```python
from build123d import *

# Parameters (mm, degrees)
SKETCH1_W           = 71.6
SKETCH1_H           = 161
SKETCH1_W_2         = 68
SKETCH1_H_2         = 30.04
BOSS_EXTRUDE1_DEPTH = 1.8
SKETCH1_6_W         = 71.6
SKETCH1_6_H         = 161
SKETCH1_6_W_2       = 68
SKETCH1_6_H_2       = 30.04
BOSS_EXTRUDE2_DEPTH = 20.1
FILLET3_SIZE        = 15
FILLET3_SIZE_2      = 10
FILLET4_R           = 15
FILLET5_SIZE        = 20
FILLET5_SIZE_2      = 15
FILLET6_SIZE        = 10
FILLET6_SIZE_2      = 15
FILLET7_SIZE        = 10
FILLET7_SIZE_2      = 15


with BuildPart() as part:
    # Sketch1 → Boss-Extrude1 (new body)
    # profile 1 of 6: a face of its own
    with BuildSketch(Plane(origin=(0, 0, 0), x_dir=(1, 0, 0), z_dir=(0, 1, 0))):
        with Locations((35.8, 80.5)):
            Rectangle(SKETCH1_W, SKETCH1_H)
        with Locations((35.8, 48.66)):
            Rectangle(SKETCH1_W_2, SKETCH1_H_2, mode=Mode.SUBTRACT)
        with Locations((35.8, 16.82)):
            Rectangle(SKETCH1_W_2, SKETCH1_H_2, mode=Mode.SUBTRACT)
        with Locations((35.8, 80.5)):
            Rectangle(SKETCH1_W_2, SKETCH1_H_2, mode=Mode.SUBTRACT)
        with Locations((35.8, 112.34)):
            Rectangle(SKETCH1_W_2, SKETCH1_H_2, mode=Mode.SUBTRACT)
        with Locations((35.8, 144.18)):
            Rectangle(SKETCH1_W_2, SKETCH1_H_2, mode=Mode.SUBTRACT)
    # profile 2 of 6: a face of its own
    with BuildSketch(Plane(origin=(0, 0, 0), x_dir=(1, 0, 0), z_dir=(0, 1, 0))):
        with Locations((35.8, 144.18)):
            Rectangle(SKETCH1_W_2, SKETCH1_H_2)
    # profile 3 of 6: a face of its own
    with BuildSketch(Plane(origin=(0, 0, 0), x_dir=(1, 0, 0), z_dir=(0, 1, 0))):
        with Locations((35.8, 112.34)):
            Rectangle(SKETCH1_W_2, SKETCH1_H_2)
    # profile 4 of 6: a face of its own
    with BuildSketch(Plane(origin=(0, 0, 0), x_dir=(1, 0, 0), z_dir=(0, 1, 0))):
        with Locations((35.8, 80.5)):
            Rectangle(SKETCH1_W_2, SKETCH1_H_2)
    # profile 5 of 6: a face of its own
    with BuildSketch(Plane(origin=(0, 0, 0), x_dir=(1, 0, 0), z_dir=(0, 1, 0))):
        with Locations((35.8, 48.66)):
            Rectangle(SKETCH1_W_2, SKETCH1_H_2)
    # profile 6 of 6: a face of its own
    with BuildSketch(Plane(origin=(0, 0, 0), x_dir=(1, 0, 0), z_dir=(0, 1, 0))):
        with Locations((35.8, 16.82)):
            Rectangle(SKETCH1_W_2, SKETCH1_H_2)
    extrude(amount=-BOSS_EXTRUDE1_DEPTH)

    # Sketch1<6> → Boss-Extrude2 (add)
    with BuildSketch(Plane(origin=(0, 0, 0), x_dir=(1, 0, 0), z_dir=(0, 1, 0))):
        with Locations((35.8, 80.5)):
            Rectangle(SKETCH1_6_W, SKETCH1_6_H)
        with Locations((35.8, 16.82)):
            Rectangle(SKETCH1_6_W_2, SKETCH1_6_H_2, mode=Mode.SUBTRACT)
        with Locations((35.8, 80.5)):
            Rectangle(SKETCH1_6_W_2, SKETCH1_6_H_2, mode=Mode.SUBTRACT)
        with Locations((35.8, 48.66)):
            Rectangle(SKETCH1_6_W_2, SKETCH1_6_H_2, mode=Mode.SUBTRACT)
        with Locations((35.8, 112.34)):
            Rectangle(SKETCH1_6_W_2, SKETCH1_6_H_2, mode=Mode.SUBTRACT)
        with Locations((35.8, 144.18)):
            Rectangle(SKETCH1_6_W_2, SKETCH1_6_H_2, mode=Mode.SUBTRACT)
    extrude(amount=BOSS_EXTRUDE2_DEPTH)

    # Fillet3
    # an asymmetric fillet: 15, 10 mm, written as the material it adds along each edge
    with BuildSketch(Plane(origin=(69.8, 0, -159.2), x_dir=(0, 1, 0), z_dir=(0, 0, 1))) as fillet3_piece_1_section:
        with BuildLine():
            Bezier((FILLET3_SIZE, 0), (0, 0), (0, FILLET3_SIZE_2), weights=[1, 0.707106781, 1])
            Line((0, FILLET3_SIZE_2), (0, 0))
            Line((0, 0), (FILLET3_SIZE, 0))
        make_face()
    fillet3_piece_1 = extrude(amount=67.54, mode=Mode.PRIVATE)
    fillet3_piece_1 = split(fillet3_piece_1, bisect_by=Plane(origin=(67.566321176, 3.350519055, -127.36), z_dir=(0, 0, -1)), keep=Keep.TOP, mode=Mode.PRIVATE)
    add(fillet3_piece_1)

    # Fillet4
    fillet4_edges = [part.edges().sort_by_distance(p)[0] for p in [
        (69.8, 0, -112.34),
    ]]
    fillet(fillet4_edges, radius=FILLET4_R)

    # Fillet5
    # an asymmetric fillet: 20, 15 mm, written as the material it adds along each edge
    with BuildSketch(Plane(origin=(69.8, 0, -95.52), x_dir=(0, 1, 0), z_dir=(0, 0, 1))) as fillet5_piece_1_section:
        with BuildLine():
            Bezier((FILLET5_SIZE, 0), (0, 0), (0, FILLET5_SIZE_2), weights=[1, 0.707106781, 1])
            Line((0, FILLET5_SIZE_2), (0, 0))
            Line((0, 0), (FILLET5_SIZE, 0))
        make_face()
    fillet5_piece_1 = extrude(amount=80.04, mode=Mode.PRIVATE)
    fillet5_piece_1 = split(fillet5_piece_1, bisect_by=Plane(origin=(69.753885797, 17.321244921, -63.68), z_dir=(0, 0, -1)), keep=Keep.TOP, mode=Mode.PRIVATE)
    add(fillet5_piece_1)

    # Fillet6
    # an asymmetric fillet: 15, 10 mm, written as the material it adds along each edge
    with BuildSketch(Plane(origin=(1.8, 0, -101.18), x_dir=(1, 0, 0), z_dir=(0, 0, 1))) as fillet6_piece_1_section:
        with BuildLine():
            Bezier((FILLET6_SIZE, 0), (0, 0), (0, FILLET6_SIZE_2), weights=[1, 0.707106781, 1])
            Line((0, FILLET6_SIZE_2), (0, 0))
            Line((0, 0), (FILLET6_SIZE, 0))
        make_face()
    fillet6_piece_1 = extrude(amount=105.04, mode=Mode.PRIVATE)
    fillet6_piece_1 = split(fillet6_piece_1, bisect_by=Plane(origin=(4.033678617, 3.350518679, -31.84), z_dir=(0, 0, -1)), keep=Keep.TOP, mode=Mode.PRIVATE)
    fillet6_piece_1 = split(fillet6_piece_1, bisect_by=Plane(origin=(4.033678617, 3.350518679, -65.48), z_dir=(0, 0, 1)), keep=Keep.TOP, mode=Mode.PRIVATE)
    add(fillet6_piece_1)

    # Fillet7
    # an asymmetric fillet: 15, 10 mm, written as the material it adds along each edge
    with BuildSketch(Plane(origin=(69.8, 0, 3.86), x_dir=(-1, 0, 0), z_dir=(0, 0, -1))) as fillet7_piece_1_section:
        with BuildLine():
            Bezier((FILLET7_SIZE, 0), (0, 0), (0, FILLET7_SIZE_2), weights=[1, 0.707106781, 1])
            Line((0, FILLET7_SIZE_2), (0, 0))
            Line((0, 0), (FILLET7_SIZE, 0))
        make_face()
    fillet7_piece_1 = extrude(amount=105.04, mode=Mode.PRIVATE)
    fillet7_piece_1 = split(fillet7_piece_1, bisect_by=Plane(origin=(67.566321383, 3.350518679, -31.84), z_dir=(0, 0, -1)), keep=Keep.TOP, mode=Mode.PRIVATE)
    add(fillet7_piece_1)


solid = part.part
```
Source: CAD feature listing. Evaluate the final solid. Frame: model axes, mm. Coordinates: 2 decimals unless noted, no trailing zeros. Loops run counter-clockwise (first coordinate to the right, second up) from the corner with the lowest first, then second, coordinate; pieces in that order, holes last. Notation, with made-up numbers: M -3,-21.75 L 18,-21.75 A26 cw 18,-5.75 Z; hole C -24,-9.75 d10. An arc over 180 degrees is marked long. Use a Markdown table: item, result. Add a question column.
Q1. Section query C-C, the plane y = 13.5. State how many separate pieces and enclosed holes the cut face has, and give its area (3 significant figures).
Q2. Material intervals for L1, parallel to Z at x = 54.5, y = 3; L2, parallel to X at y = 14.5, z = -152; L3, parallel to Z at x = 5, y = 3, sorted ascending.
Q3. Draft query along Z for faces 1 (the flat face through (69.8, 18, -48)), 2 (the flat face through (35, 9, 0)), 3 (the flat face through (1, 20.1, -81)), 4 (the flat face through (35, 9, -161)). Return one class per face: pulls with the +Z half, pulls with the -Z half, needs draft (parallel to the pull), parting line crosses it, or undercut.
Q4. First-contact query: pin 1 (4 mm diameter, centred on x = 40, z = -59.5, fed in from +Y). Flat tip, straight axial feed; report the tip coordinate or a pass-through.
Q5. Section query A-A, the plane z = -122.5. Return loops of the section in (x, y), and give its area (3 significant figures).
Q6. Section query B-B, the plane x = 18.5. Return loops of the section in (y, z), and give its area (3 significant figures).
Result:
| question | item | result |
|---|---|---|
| 1 | separate pieces | 1 |
| 1 | enclosed holes | 5 |
| 1 | area | 1,350 mm2 |
| 2 | L1 | z = -161 to -159.2, -129.16 to -127.36, -97.32 to -95.52, -65.48 to -63.68, -33.64 to -31.84, -1.8 to 0 |
| 2 | L2 | x = 0 to 1.8, 69.79 to 71.6 |
| 2 | L3 | z = -161 to -159.2, -129.16 to -127.36, -97.32 to -95.52, -65.48 to -31.84, -1.8 to 0 |
| 3 | face 1 | undercut |
| 3 | face 2 | pulls with the +Z half |
| 3 | face 3 | needs draft |
| 3 | face 4 | pulls with the -Z half |
| 4 | pin 1 | stops at y = 0 |
| 5 | outline | M 0,-1.8 L 71.6,-1.8 L 71.6,20.1 L 69.8,20.1 L 69.8,15 A15 cw 54.8,0 L 1.8,0 L 1.8,20.1 L 0,20.1 Z |
| 5 | area | 250 mm2 |
| 6 | outline | M -1.8,-161 L 20.1,-161 L 20.1,-159.2 L 0,-159.2 L 0,-129.16 L 20.1,-129.16 L 20.1,-127.36 L 0,-127.36 L 0,-97.32 L 20.1,-97.32 L 20.1,-95.52 L 0,-95.52 L 0,-65.48 L 20.1,-65.48 L 20.1,-63.68 L 0,-63.68 L 0,-33.64 L 20.1,-33.64 L 20.1,-31.84 L 0,-31.84 L 0,-1.8 L 20.1,-1.8 L 20.1,0 L -1.8,0 Z |
| 6 | area | 507 mm2 |
